from build123d import *

# Parameters (mm, degrees)
SKETCH2_R           = 9
SKETCH2_R_2         = 4
SKETCH2_R_3         = 3.175
BOSS_EXTRUDE1_DEPTH = 31.75
CUT_EXTRUDE7_DEPTH  = 19.05
SKETCH4_R           = 11
CUT_EXTRUDE8_DEPTH  = 18.875
SKETCH5_R           = 11.825
CUT_EXTRUDE9_DEPTH  = 1.2


with BuildPart() as part:
    # Sketch2 → Boss-Extrude1 (new body)
    with BuildSketch(Plane(origin=(0, 0, 0), x_dir=(1, 0, 0), z_dir=(0, 1, 0))):
        with BuildLine():
            Line((16.780050899, 23.273406552), (76.169078327, 0.999356152))
            ThreePointArc((76.169078327, 0.999356152), (83.295947219, 0.081549283), (90.085976392, 2.43317287))
            Line((90.085976392, 2.43317287), (116.795312979, 19.333283493))
            ThreePointArc((116.795312979, 19.333283493), (122.299175659, 33.248981014), (110.733053142, 42.744451083))
            Line((110.733053142, 42.744451083), (21.968243349, 47.843674862))
            ThreePointArc((21.968243349, 47.843674862), (8.8138749, 37.788419678), (16.780050899, 23.273406552))
        make_face()
        with Locations((81.685914874, 15.708829783)):
            Circle(SKETCH2_R, mode=Mode.SUBTRACT)
        with Locations((110.004683999, 30.065354964)):
            Circle(SKETCH2_R_2, mode=Mode.SUBTRACT)
        with Locations((21.239874206, 35.164578743)):
            Circle(SKETCH2_R_2, mode=Mode.SUBTRACT)
        with Locations((50, 35.164578743)):
            Circle(SKETCH2_R_3, mode=Mode.SUBTRACT)
    extrude(amount=-BOSS_EXTRUDE1_DEPTH)

    # Sketch3 → Cut-Extrude7 (cut)
    with BuildSketch(Plane(origin=(0, -6.35, 0), x_dir=(1, 0, 0), z_dir=(0, 1, 0))):
        with BuildLine():
            Line((94.910034212, 24.187626921), (101.811056049, 13.424315235))
            ThreePointArc((101.811056049, 13.424315235), (102.214392091, 11.155436631), (100.889566337, 9.269879207))
            Line((100.889566337, 9.269879207), (124.896489339, 9.269879207))
            Line((124.896489339, 9.269879207), (123.850468237, 47.864578743))
            Line((123.850468237, 47.864578743), (8.539874206, 47.864578743))
            Line((8.539874206, 47.864578743), (8.539874206, 20.980420685))
            Line((8.539874206, 20.980420685), (64.646726928, 5.321032632))
            ThreePointArc((64.646726928, 5.321032632), (63.234252728, 6.421229435), (62.7, 8.130056632))
            Line((62.7, 8.130056632), (62.7, 18.708063959))
            ThreePointArc((62.7, 18.708063959), (62.972728913, 19.95786091), (63.741328279, 20.980420685))
            Line((63.741328279, 20.980420685), (71.429767985, 27.607518121))
            ThreePointArc((71.429767985, 27.607518121), (83.950010515, 31.253642555), (94.910034212, 24.187626921))
        make_face()
    extrude(amount=-CUT_EXTRUDE7_DEPTH, mode=Mode.SUBTRACT)

    # Sketch4 → Cut-Extrude8 (cut)
    with BuildSketch(Plane(origin=(0, 0, 0), x_dir=(1, 0, 0), z_dir=(0, 1, 0))):
        with Locations((81.685914874, 15.708829783)):
            Circle(SKETCH4_R)
    extrude(amount=-CUT_EXTRUDE8_DEPTH, mode=Mode.SUBTRACT)

    # Sketch5 → Cut-Extrude9 (cut)
    with BuildSketch(Plane(origin=(0, -12.875, 0), x_dir=(1, 0, 0), z_dir=(0, 1, 0))):
        with Locations((81.685914874, 15.708829783)):
            Circle(SKETCH5_R)
    extrude(amount=CUT_EXTRUDE9_DEPTH, mode=Mode.SUBTRACT)


solid = part.part
Work out the finished part from the listing and answer in its coordinate system (mm). A direction names the side the tool comes from. Round coordinates to 2 decimals unless told otherwise and drop trailing zeros. Loops run counter-clockwise (first coordinate to the right, second up) from the corner with the lowest first, then second, coordinate; pieces in that order, holes last. Notation, with made-up numbers: M -38.5,4.25 L -19.5,4.25 A23 ccw -19.5,26.25 Z; hole C -9,-21 d5. An arc over 180 degrees is marked long. One line per question, with ' | ' between items. Start each with the question number.
(1) A cutting plane is placed at D-D on z = -17. Write down the section's boundary in (x, y) (3 decimals), plus the area to 3 significant figures.
(2) Flat-ended cylindrical pins translate along their axes: pin 1 Ø4 at (x, y) = (68, -23.5) entering from -Z; pin 2 Ø6.5 at (x, z) = (21.24, -35.16) entering from -Y; pin 3 Ø8.5 at (y, z) = (-11, -14.5) entering from -X; pin 4 Ø5 at (y, z) = (-9, -22) entering from -X. Find the tip coordinate at first contact, or state that the pin passes through.
(3) A cutting plane is placed at B-B on x = 86. Write down the section's boundary in (y, z) (3 decimals), plus the area to 3 significant figures.
(4) A tool of negligible diameter and unlimited length cuts with its end or side. For faces 5 (the face through (80.254, -5.756, -26.615)), 6 (the face through (83.76, -15.74, -31.28)), 7 (the face through (63.25, -15.74, -6.4)), 8 (the face through (85, -12.875, -5)), from which of +Z, -Z, +X, -X, +Y, -Y can it reach the whole face along a straight path? Write none if from no direction.
(5) Find the intervals of material crossed by line 1 (Y direction, x = 39, z = -23); line 2 (X direction, y = -12, z = -22); line 3 (Z direction, x = 77, y = -6), in increasing order.
(6) For a pull along Z with two mould halves and no side action, classify faces 1 (the face through (65, -25.4, -32)), 2 (the face through (52.7, -5.1, -9.8)), 3 (the face through (62.965, -15.742, -19.941)), 4 (the face through (106.01, -3.13, -30.24)) as released by +Z, released by -Z, zero draft, split by the parting line, or undercut.
(7) A cutting plane is placed at A-A on x = 50. Write down the section's boundary in (y, z).
Geometry check:
1) outline: M 33.507,-31.75 L 72.779,-31.75 L 72.779,-18.875 L 70.762,-18.875 L 70.762,-12.875 L 69.932,-12.875 L 69.932,-11.675 L 70.762,-11.675 L 70.762,0 L 33.507,0 L 33.507,-6.35 L 62.7,-6.35 L 62.7,-25.4 L 33.507,-25.4 Z; M 90.593,-31.75 L 113.108,-31.75 L 113.108,-25.4 L 99.518,-25.4 L 99.518,-6.35 L 113.108,-6.35 L 113.108,0 L 92.61,0 L 92.61,-11.675 L 93.44,-11.675 L 93.44,-12.875 L 92.61,-12.875 L 92.61,-18.875 L 90.593,-18.875 Z | area: 1,070 mm²
2) pin 1: stops at z = -45.24 | pin 2: passes through | pin 3: stops at x = 62.7 | pin 4: stops at x = 62.81
3) outline: M -31.75,-44.165 L -25.4,-44.165 L -25.4,-30.814 L -6.35,-30.814 L -6.35,-44.165 L 0,-44.165 L 0,-25.828 L -11.675,-25.828 L -11.675,-26.719 L -12.875,-26.719 L -12.875,-25.828 L -18.875,-25.828 L -18.875,-23.607 L -31.75,-23.607 Z; M -31.75,-7.81 L -18.875,-7.81 L -18.875,-5.59 L -12.875,-5.59 L -12.875,-4.699 L -11.675,-4.699 L -11.675,-5.59 L 0,-5.59 L 0,-0.603 L -31.75,-0.603 Z | area: 541 mm²
4) face 5: +Y | face 6: -Z | face 7: +Z, -X | face 8: none
5) line 1: y = -31.75 to -25.4, -6.35 to 0 | line 2: x = 64.92 to 71.67, 91.7 to 96.31 | line 3: z = -44.68 to -25.66, -5.76 to -0.71
6) face 1: zero draft | face 2: released by +Z | face 3: released by -Z | face 4: undercut
7) outline: M -31.75,-46.23 L -25.4,-46.23 L -25.4,-38.34 L -31.75,-38.34 Z; M -31.75,-31.99 L -25.4,-31.99 L -25.4,-10.81 L -31.75,-10.81 Z; M -6.35,-46.23 L 0,-46.23 L 0,-38.34 L -6.35,-38.34 Z; M -6.35,-31.99 L 0,-31.99 L 0,-10.81 L -6.35,-10.81 Z
